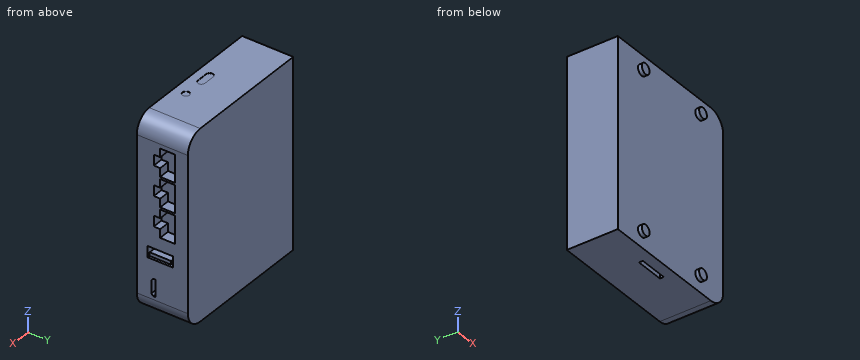
from build123d import *

# Parameters (mm, degrees)
ESQUISSE1_W             = 68
ESQUISSE1_H             = 88.6
BOSS_EXTRU_1_DEPTH      = 24
ESQUISSE2_W             = 5.2
ESQUISSE2_H             = 12
ESQUISSE2_W_2           = 1.7
ESQUISSE2_H_2           = 10
ENL_V_MAT_EXTRU_1_DEPTH = 5
ESQUISSE3_W             = 13.5
ESQUISSE3_H             = 1.8
ENL_V_MAT_EXTRU_2_DEPTH = 5
ESQUISSE4_R             = 1.65
ENL_V_MAT_EXTRU_3_DEPTH = 0.1
ESQUISSE5_R             = 2.5
BOSS_EXTRU_3_DEPTH      = 1.8
CONG_1_R                = 8


with BuildPart() as part:
    # Esquisse1 → Boss.-Extru.1 (new body)
    with BuildSketch(Plane(origin=(0, 0, 0), x_dir=(1, 0, 0), z_dir=(0, 1, 0))):
        Rectangle(ESQUISSE1_W, ESQUISSE1_H)
    extrude(amount=BOSS_EXTRU_1_DEPTH)

    # Esquisse2 → Enlèv. mat.-Extru.1 (cut)
    # profile 1 of 5: a face of its own
    with BuildSketch(Plane(origin=(34, 0, 0), x_dir=(0, 0, -1), z_dir=(1, 0, 0))):
        Polygon((-34.3, 18), (-34.3, 11), (-30.3, 11), (-30.3, 8), (-25.3, 8), (-25.3, 11), (-21.3, 11), (-21.3, 18), align=None)
    # profile 2 of 5: a face of its own
    with BuildSketch(Plane(origin=(34, 0, 0), x_dir=(0, 0, -1), z_dir=(1, 0, 0))):
        Polygon((-7.3, 18), (-20.3, 18), (-20.3, 11), (-16.3, 11), (-16.3, 8), (-11.3, 8), (-11.3, 11), (-7.3, 11), align=None)
    # profile 3 of 5: a face of its own
    with BuildSketch(Plane(origin=(34, 0, 0), x_dir=(0, 0, -1), z_dir=(1, 0, 0))):
        Polygon((6.7, 18), (-6.3, 18), (-6.3, 11), (-2.3, 11), (-2.3, 8), (2.7, 8), (2.7, 11), (6.7, 11), align=None)
    # profile 4 of 5: a face of its own
    with BuildSketch(Plane(origin=(34, 0, 0), x_dir=(0, 0, -1), z_dir=(1, 0, 0))):
        Polygon((26.784034195, 8.864890508), (34.784034195, 8.864890508), (34.784034195, 7.653311673), (33.810896432, 6.864890508), (27.757171958, 6.864890508), (26.784034195, 7.653311673), align=None)
    # profile 5 of 5: a face of its own
    with BuildSketch(Plane(origin=(34, 0, 0), x_dir=(0, 0, -1), z_dir=(1, 0, 0))):
        with Locations((15.369525707, 11.07791291)):
            Rectangle(ESQUISSE2_W, ESQUISSE2_H)
        with Locations((16.119525707, 11.07791291)):
            Rectangle(ESQUISSE2_W_2, ESQUISSE2_H_2, mode=Mode.SUBTRACT)
    extrude(amount=-ENL_V_MAT_EXTRU_1_DEPTH, mode=Mode.SUBTRACT)

    # Esquisse3 → Enlèv. mat.-Extru.2 (cut)
    with BuildSketch(Plane(origin=(0, 0, -44.3), x_dir=(-1, 0, 0), z_dir=(0, 0, -1))):
        with Locations((4.25, 5.9)):
            Rectangle(ESQUISSE3_W, ESQUISSE3_H)
    extrude(amount=-ENL_V_MAT_EXTRU_2_DEPTH, mode=Mode.SUBTRACT)

    # Esquisse4 → Enlèv. mat.-Extru.3 (cut)
    with BuildSketch(Plane.XY.offset(44.3)):
        with Locations((10.211694525, 5.763285302)):
            Circle(ESQUISSE4_R)
        with BuildLine():
            Line((-5.15123343, 7.413285302), (0.211694525, 7.413285302))
            ThreePointArc((0.211694525, 7.413285302), (1.861694525, 5.763285302), (0.211694525, 4.113285302))
            Line((0.211694525, 4.113285302), (-5.15123343, 4.113285302))
            ThreePointArc((-5.15123343, 4.113285302), (-6.80123343, 5.763285302), (-5.15123343, 7.413285302))
        make_face()
    extrude(amount=-ENL_V_MAT_EXTRU_3_DEPTH, mode=Mode.SUBTRACT)

    # Esquisse5 → Boss.-Extru.3 (add)
    with BuildSketch(Plane.XZ):
        with Locations(Location((-18.5, 37, 0), (0, 0, 90))):
            Circle(ESQUISSE5_R)
        with Locations(Location((18.5, 37, 0), (0, 0, 90))):
            Circle(ESQUISSE5_R)
        with Locations(Location((18.5, -37, 0), (0, 0, 90))):
            Circle(ESQUISSE5_R)
        with Locations(Location((-18.5, -37, 0), (0, 0, 90))):
            Circle(ESQUISSE5_R)
    extrude(amount=BOSS_EXTRU_3_DEPTH)

    # Congé1
    cong_1_edges = [part.edges().sort_by_distance(p)[0] for p in [
        (34, 12, -44.3),
        (34, 12, 44.3),
    ]]
    fillet(cong_1_edges, radius=CONG_1_R)


solid = part.part
Can you work these out from the model? Positions are in its coordinate system, mm. Coordinates: 2 decimals unless noted, no trailing zeros. Loops run counter-clockwise (first coordinate to the right, second up) from the corner with the lowest first, then second, coordinate; pieces in that order, holes last. Notation, with made-up numbers: (82.5, -5) - (139.5, -5) arc R22 ccw to (139.5, 13) - close; hole circle Ø10 at (-12.5, 54.5). An arc over 180 degrees is marked (long way). Put each result on its own line as item: value. Start each with the question number.
Item 1: Suppose I cut it at D-D (z = -0.5). Please give me the cut outline in (x, y), and give its area (3 significant figures).
Item 2: Suppose I cut it at A-A (x = -20). Please give me the cut outline in (y, z), and give its area (3 significant figures).
Item 3: Suppose I cut it at C-C (y = 10). Please give me the cut outline in (x, z), and give its area (3 significant figures).
Item 4: For pin 1 (4 mm diameter, centred on x = -23, z = -1.5, fed in from -Y); pin 2 (2.5 mm diameter, centred on x = -2.5, y = 5, fed in from +Z); pin 3 (1.5 mm diameter, centred on x = 30.5, y = 9, fed in from -Z); pin 4 (5.5 mm diameter, centred on x = 31, y = 10.5, fed in from +Z), each with a flat end and sliding along its axis, tell me the tip position at first contact or that it passes through.
Item 5: If I drill on line 1 along Y through (x, z) = (-19, -18); line 2 along X through (y, z) = (10, -36.5); line 3 along X through (y, z) = (11.25, -2), over which ranges is the centre line in solid material (lowest first)?
Item 6: Suppose I cut it at B-B (z = -14). Please give me the cut outline in (x, y), and give its area (3 significant figures).
Here are the results:
1. outline: (-34, 0) - (34, 0) - (34, 8) - (29, 8) - (29, 18) - (34, 18) - (34, 24) - (-34, 24) - close
1. area: 1,580 mm²
2. outline: (-1.8, -39) - (0, -39) - (0, -44.3) - (24, -44.3) - (24, 44.3) - (0, 44.3) - (0, 39) - (-1.8, 39) - (-1.8, 35) - (0, 35) - (0, -35) - (-1.8, -35) - close
2. area: 2,140 mm²
3. outline: (-34, -44.3) - (26, -44.3) arc R8 ccw to (34, -36.3) - (34, -17.97) - (29, -17.97) - (29, -16.97) - (34, -16.97) - (34, -15.27) - (29, -15.27) - (29, -12.77) - (34, -12.77) - (34, -2.7) - (29, -2.7) - (29, 2.3) - (34, 2.3) - (34, 11.3) - (29, 11.3) - (29, 16.3) - (34, 16.3) - (34, 25.3) - (29, 25.3) - (29, 30.3) - (34, 30.3) - (34, 36.3) arc R8 ccw to (26, 44.3) - (-34, 44.3) - close
3. area: 5,900 mm²
4. pin 1: y = 0
4. pin 2: z = 44.3
4. pin 3: z = -43.37
4. pin 4: z = 43.98
5. line 1: 0 to 24
5. line 2: -34 to 34
5. line 3: -34 to 29
6. outline: (-34, 0) - (34, 0) - (34, 5.08) - (29, 5.08) - (29, 17.08) - (34, 17.08) - (34, 24) - (-34, 24) - close
6. area: 1,570 mm²
